Model file for the job. Use its own axes, mm. A direction names the side the tool comes from. Coordinates: 2 decimals unless noted, no trailing zeros. Order: outer loops, then holes, each group sorted by start corner. A loop starts at its lowest first (then second) coordinate and runs counter-clockwise, first axis right, second up. Notation, with made-up numbers: (52, 28) -> (101, 28) arc R13 cw to (101, 50) -> close; hole circle Ø3 at (-2.5, 51.25). An arc over 180 degrees is marked (long way). Write item = value, one per line. Start each with the question number.
Q1. Cut at A-A, the plane x = -5. List the corners of the cut face in (y, z) (1 decimal), plus the area to 3 significant figures.
Q2. Cut at C-C, the plane x = 17. List the corners of the cut face in (y, z).
Q3. Wall check: line 1 (Z direction, x = -8, y = 18); line 2 (X direction, y = -5, z = -18); line 3 (Y direction, x = -14.5, z = -22). Give the ranges that are in metal, low to high. Write a range as from..to.
Q4. Flat gauge pins, fed straight in: pin 1 (6 mm diameter, centred on y = 3, z = -9.5, fed in from -X); pin 2 (5 mm diameter, centred on y = -21, z = -18.5, fed in from -X); pin 3 (1.5 mm diameter, centred on x = -15, z = -20, fed in from -Y); pin 4 (15.5 mm diameter, centred on y = 0, z = 0, fed in from +X). Where does each tip first touch, or does it go through?
Q5. 3-axis set-ups, long thin cutter, end or side, ignore diameter. For faces 1 (the face through (-6, 1, -24)), 2 (the face through (-4.03, 21.97, 7.41)), 3 (the face through (-6.1, -16.8, -19.7)), 4 (the face through (-20.4, -6, -18)): which of +Z, -Z, +X, -X, +Y, -Y reach the whole face in a straight line?
Q6. Mould opens along X. For faces 5 (the face through (-23, 6, -18)), 6 (the face through (4, 20, 20)), 7 (the face through (-6.1, 19.7, -16.8)) say: +X half, -X half, draft (parallel to the pull), parting line (faces both ways), or undercut.
Q7. Cut at B-B, the plane x = -15. List the corners of the cut face in (y, z), plus the area to 3 significant figures.
Q8. Cut at D-D, the plane z = -4. Give the number of separate pieces and of enclosed holes in the cut face, plus the area to 3 significant figures.
from build123d import *

# Parameters (mm, degrees)
ESQUISSE2_W                  = 51
ESQUISSE2_H                  = 6
ENL_V_MAT_EXTRU_1_DEPTH      = 25
ENL_V_MAT_EXTRU_2_REACH      = 70
ESQUISSE3_R                  = 7.475
ESQUISSE4_R                  = 3
ENL_V_MAT_EXTRU_3_DEPTH      = 20
R_P_TITION_CIRCULAIRE1_COUNT = 4
ESQUISSE7_R                  = 3
ENL_V_MAT_EXTRU_5_DEPTH      = 11
ENL_V_MAT_EXTRU_6_REACH      = 61
ESQUISSE8_R                  = 1


with BuildPart() as part:
    # Esquisse1 → Base-Révolution (revolve)
    with BuildSketch(Plane.XY):
        Polygon((-26, 16), (-26, 20), (-23, 20), (-23, 18.5), (-20.4, 18.5), (-20.4, 20), (-16, 20), (-16, 35), (6, 35), (21, 20), (21, 10), (18, 10), (18, 13.25), (14, 13.25), (14, 10), (3.732050808, 10), (2, 13), (-23, 13), align=None)
    revolve(axis=Axis((-21, 0, 0), (1, 0, 0)))

    # Esquisse2 → Enlèv. mat.-Extru.1 (cut, symmetric)
    with BuildSketch(Plane.XY):
        with Locations((-5.5, 36)):
            Rectangle(ESQUISSE2_W, ESQUISSE2_H)
    extrude(amount=ENL_V_MAT_EXTRU_1_DEPTH, both=True, mode=Mode.SUBTRACT)

    # Esquisse3 → Enlèv. mat.-Extru.2 (cut, up to next)
    with BuildSketch(Plane(origin=(0, 33, 0), x_dir=(-1, 0, 0), z_dir=(0, 1, 0)), mode=Mode.PRIVATE) as enl_v_mat_extru_2_sk1:
        with Locations((5, 0)):
            Circle(ESQUISSE3_R)
    enl_v_mat_extru_2_tool1 = extrude(enl_v_mat_extru_2_sk1.sketch, amount=-ENL_V_MAT_EXTRU_2_REACH, mode=Mode.PRIVATE) & part.part
    add(enl_v_mat_extru_2_tool1.solids().sort_by_distance((-5, 33, 0))[0], mode=Mode.SUBTRACT)

    # Esquisse4 → Enlèv. mat.-Extru.3 (cut)
    with BuildSketch(Plane.ZY.offset(16)):
        with Locations((19.798989873, -19.798989873)):
            Circle(ESQUISSE4_R)
    enl_v_mat_extru_3 = extrude(amount=-ENL_V_MAT_EXTRU_3_DEPTH, mode=Mode.SUBTRACT)

    # Répétition circulaire1: Enlèv. mat.-Extru.3 ×4 about axis
    r_p_tition_circulaire1_axis = Axis((-21, 0, 0), (1, 0, 0))
    for i in range(1, R_P_TITION_CIRCULAIRE1_COUNT):
        add(enl_v_mat_extru_3.rotate(r_p_tition_circulaire1_axis, i * 360 / R_P_TITION_CIRCULAIRE1_COUNT), mode=Mode.SUBTRACT)

    # Esquisse7 → Enlèv. mat.-Extru.5 (cut)
    with BuildSketch(Plane.XY.offset(-35)):
        with Locations((-5, 0.349567503)):
            Circle(ESQUISSE7_R)
    extrude(amount=ENL_V_MAT_EXTRU_5_DEPTH, mode=Mode.SUBTRACT)

    # Esquisse8 → Enlèv. mat.-Extru.6 (cut, up to next)
    with BuildSketch(Plane(origin=(0, 0, -24), x_dir=(-1, 0, 0), z_dir=(0, 0, -1)), mode=Mode.PRIVATE) as enl_v_mat_extru_6_sk1:
        with Locations((5, 0.349567503)):
            Circle(ESQUISSE8_R)
    enl_v_mat_extru_6_tool1 = extrude(enl_v_mat_extru_6_sk1.sketch, amount=-ENL_V_MAT_EXTRU_6_REACH, mode=Mode.PRIVATE) & part.part
    add(enl_v_mat_extru_6_tool1.solids().sort_by_distance((-5, 0.349568, -24))[0], mode=Mode.SUBTRACT)


solid = part.part
Here are the results:
q1.outline = (-2.7, -34.9) -> (-2.7, -24) -> (-0.7, -24) -> (-0.7, -13) arc R13 cw (long way) to (10.6, 7.5) -> (33, 7.5) -> (33, 11.7) arc R35 ccw (long way) to start; (1.3, -24) -> (3.3, -24) -> (3.3, -34.8) arc R35 ccw to (33, -11.7) -> (33, -7.5) -> (10.6, -7.5) arc R13 cw to (1.3, -12.9) -> close; hole circle Ø6 at (-19.8, -19.8); hole circle Ø6 at (-19.8, 19.8); hole circle Ø6 at (19.8, -19.8); hole circle Ø6 at (19.8, 19.8)
q1.area = 2,780 mm²
q2.outline = circle Ø48 at (0, 0); hole circle Ø26.5 at (0, 0)
q3.line_1 = -30.02..-22.2, -17.4..-6.85, 6.85..17.4, 22.2..30.02
q3.line_2 = -26..-23, -20.4..21
q3.line_3 = -27.22..-21.84, -17.76..17.76, 21.84..27.22
q4.pin_1 = 2.02
q4.pin_2 = -16
q4.pin_3 = -29.23
q4.pin_4 = through
q5.face_1 = -Z
q5.face_2 = +Y
q5.face_3 = -X
q5.face_4 = none
q6.face_5 = undercut
q6.face_6 = -X half
q6.face_7 = draft
q7.outline = (33, -11.66) -> (33, 11.66) arc R35 ccw (long way) to start; hole circle Ø6 at (-19.8, -19.8); hole circle Ø6 at (-19.8, 19.8); hole circle Ø26 at (0, 0); hole circle Ø6 at (19.8, -19.8); hole circle Ø6 at (19.8, 19.8)
q7.area = 3,170 mm²
q8.separate_pieces = 3
q8.enclosed_holes = 0
q8.area = 1,350 mm²
